Part print with two shaded views. Sizes in mm from the minimum x, y, z corner. Give positions to 0.01 mm unless a question says otherwise; leave off trailing zeros. Order: outer loops, then holes, each group sorted by start corner. A loop starts at its lowest first (then second) coordinate and runs counter-clockwise, first axis right, second up. Notation, with made-up numbers: M -35,-15.75 L 24,-15.75 A27 cw 24,7.25 Z; hole C -28,66 d2. An arc over 180 degrees is marked long. Return JSON: item names as keys, results as strings. Group by question number.
1. Slice it at A-A on y = 36. List the corners of the cut face in (x, z) (1 decimal), then the cut area to 3 significant figures.
2. Pin check, flat tips, straight feed: pin 1 (6.5 mm diameter, centred on x = 51.56, y = 20.44, fed in from +Z) (3 decimals); pin 2 (4 mm diameter, centred on x = 51.56, y = 51.56, fed in from +Z). Stop position of each tip, or through.
3. Slice it at D-D on x = 62. List the corners of the cut face in (y, z) (1 decimal).
4. Wall check: probe 1 along Y at (x, z) = (36, 2.45); probe 2 along Y at (x, z) = (19, 0.3); probe 3 along Y at (x, z) = (61.5, 1.9) (1 decimal). Give the ranges that are in metal, low to high. Write a range as [from, to].
5. Slice it at C-C on y = 9. List the corners of the cut face in (x, z) (1 decimal), then the cut area to 3 significant figures.
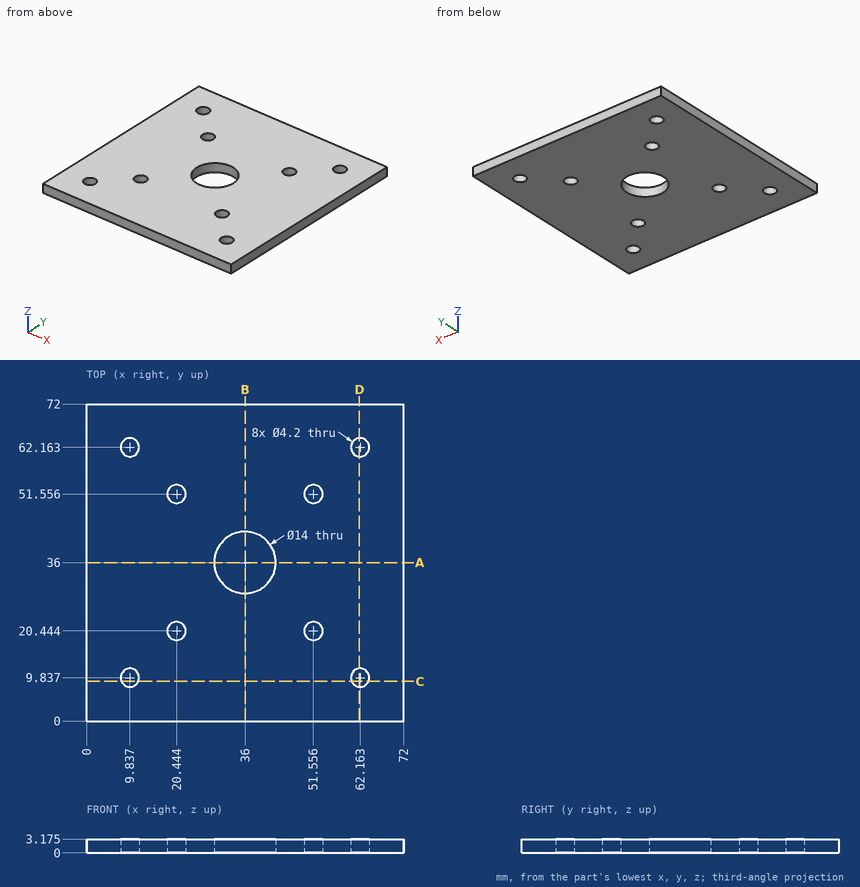
Result:
{
 "1": {"outline": "M 0,0 L 29,0 L 29,3.2 L 0,3.2 Z; M 43,0 L 72,0 L 72,3.2 L 43,3.2 Z", "area": "184 mm2"},
 "2": {"pin 1": "stops at z = 3.175", "pin 2": "passes through"},
 "3": {"outline": "M 0,0 L 7.7,0 L 7.7,3.2 L 0,3.2 Z; M 11.9,0 L 60.1,0 L 60.1,3.2 L 11.9,3.2 Z; M 64.3,0 L 72,0 L 72,3.2 L 64.3,3.2 Z"},
 "4": {"probe 1": "y = [0, 29], [43, 72]", "probe 2": "y = [0, 18.92], [21.97, 50.03], [53.08, 72]", "probe 3": "y = [0, 7.8], [11.8, 60.2], [64.2, 72]"},
 "5": {"outline": "M 0,0 L 7.9,0 L 7.9,3.2 L 0,3.2 Z; M 11.8,0 L 60.2,0 L 60.2,3.2 L 11.8,3.2 Z; M 64.1,0 L 72,0 L 72,3.2 L 64.1,3.2 Z", "area": "204 mm2"}
}
